Work out the finished part from the listing and answer in its coordinate system (mm). A direction names the side the tool comes from. Round coordinates to 2 decimals unless told otherwise and drop trailing zeros. Loops run counter-clockwise (first coordinate to the right, second up) from the corner with the lowest first, then second, coordinate; pieces in that order, holes last. Notation, with made-up numbers: (9.5, -38.75) - (15.5, -38.75) arc R17 cw to (15.5, -10.75) - close; hole circle Ø11 at (80, 16). An arc over 180 degrees is marked (long way). Answer as CSV lines item,"result". Start each with the question number.
Q1. Section B-B on x = -6 is taken. Write down the section's boundary in (y, z), then the cut area to 3 significant figures.
Q2. Section A-A on z = -1.2 is taken. Write down the section's boundary in (x, y).
Q3. Each of these flat-tipped pins is pushed along its axis until it touches: pin 1 Ø6 at (x, y) = (14, 3) entering from -Z; pin 2 Ø1 at (x, y) = (-5, 11) entering from -Z; pin 3 Ø1 at (y, z) = (32.5, -1) entering from -X; pin 4 Ø1.6 at (x, z) = (4, -1.5) entering from +Y. Where does it stop, or does it pass through?
Q4. Straight lines are drawn through the part: L1, parallel to Y at x = 12, z = -1.15; L2, parallel to Z at x = -2.5, y = 22; L3, parallel to X at y = 46.5, z = -0.4. For each, find the intervals that lie inside material, in ascending order. Write a range as [from, to].
Q5. For faces 1 (the face through (15.532, 23, -1)), 2 (the face through (2, 48, 1)), determine the directions among +Z, -Z, +X, -X, +Y, -Y from which every point of the face is accessible in a straight line to the end or side of a thin tool.
```python
from build123d import *

# Parameters (mm, degrees)
SKETCH2_W           = 27
SKETCH2_H           = 48
BOSS_EXTRUDE1_DEPTH = 2
BOSS_EXTRUDE2_DEPTH = 2


with BuildPart() as part:
    # Sketch2 → Boss-Extrude1 (new body)
    with BuildSketch(Plane.XY):
        with Locations((-0.118075802, 24)):
            Rectangle(SKETCH2_W, SKETCH2_H)
        with BuildLine():
            Line((-13.618075802, 0), (-13.618075802, -2))
            Line((-13.618075802, -2), (13.381924198, -2))
            ThreePointArc((13.381924198, -2), (14.796137761, -1.414213562), (15.381924198, 0))
            Line((15.381924198, 0), (15.381924198, 48))
            Line((15.381924198, 48), (13.381924198, 48))
            Line((13.381924198, 48), (13.381924198, 0))
            Line((13.381924198, 0), (-13.618075802, 0))
        make_face()
        Polygon((17.531924198, 48), (17.531924198, -2.15), (15.531924198, -2.15), (15.531924198, -2), (15.531924198, 48), align=None)
        Polygon((15.531924198, -2.15), (-13.618075802, -2.15), (-13.618075802, -4.15), (17.531924198, -4.15), (17.531924198, -2.15), align=None)
        with BuildLine():
            Line((15.381924198, -2), (15.381924198, 0))
            ThreePointArc((15.381924198, 0), (14.796137761, -1.414213562), (13.381924198, -2))
            Line((13.381924198, -2), (15.381924198, -2))
        make_face()
        Polygon((15.531924198, 48), (15.381924198, 48), (15.381924198, 0), (15.381924198, -2), (15.531924198, -2), align=None)
        Polygon((15.531924198, -2), (15.381924198, -2), (13.381924198, -2), (-13.618075802, -2), (-13.618075802, -2.15), (15.531924198, -2.15), align=None)
    extrude(amount=BOSS_EXTRUDE1_DEPTH)

    # Sketch2_4 → Boss-Extrude2 (add)
    with BuildSketch(Plane.XY):
        Polygon((15.531924198, -2.15), (-13.618075802, -2.15), (-13.618075802, -4.15), (17.531924198, -4.15), (17.531924198, -2.15), align=None)
        Polygon((17.531924198, 48), (17.531924198, -2.15), (15.531924198, -2.15), (15.531924198, -2), (15.531924198, 48), align=None)
    extrude(amount=-BOSS_EXTRUDE2_DEPTH)


solid = part.part
```
Findings:
1,outline,"(-4.15, -2) - (-2.15, -2) - (-2.15, 0) - (48, 0) - (48, 2) - (-4.15, 2) - close"
1,area,"108 mm^2"
2,outline,"(-13.62, -4.15) - (17.53, -4.15) - (17.53, 48) - (15.53, 48) - (15.53, -2.15) - (-13.62, -2.15) - close"
3,pin 1,"stops at z = -2"
3,pin 2,"stops at z = 0"
3,pin 3,"stops at x = 15.53"
3,pin 4,"stops at y = -2.15"
4,L1,"y = [-4.15, -2.15]"
4,L2,"z = [0, 2]"
4,L3,"x = [15.53, 17.53]"
5,face 1,"-Z, -X, +Y"
5,face 2,"+Z, -Z, +X, -X, +Y"
